Can you work these out from the model? Positions are in its coordinate system, mm. A direction names the side the tool comes from. Round coordinates to 2 decimals unless told otherwise and drop trailing zeros. Loops run counter-clockwise (first coordinate to the right, second up) from the corner with the lowest first, then second, coordinate; pieces in that order, holes last.
(1) If I drill on line 1 along Y through (x, z) = (-45, 27.75); line 2 along Y through (x, z) = (687, 2.5), over which ranges is the centre line in solid material (lowest first)?
(2) I want a section at B-B on z = 13.5. Write out the boundary of the cut face in (x, y).
(3) Will these pins go through, and if not, where does the flat tip stop? pin 1 Ø2 at (x, y) = (-8.5, 22.5) entering from +Z; pin 2 Ø0.6 at (y, z) = (40, 0.5) entering from -X; pin 3 Ø1.6 at (y, z) = (39, 0.5) entering from +X.
(4) Which directions (+Z, -Z, +X, -X, +Y, -Y) give clear straight access to the entire face, cutting with the end or side of a thin tool? Please do faces 1 (the face through (10, 2, 17)), 2 (the face through (-750, 1.6, 8.4)).
(5) I want a section at A-A on x = -250. Write out the boundary of the cut face in (y, z) (3 decimals), plus the area to 3 significant figures.
(6) I want a section at C-C on x = 462. Write out the boundary of the cut face in (y, z) (3 decimals), plus the area to 3 significant figures.
Autodesk Inventor part; units mm, degrees
ref_plane "YZ Plane" through (0, 0, 0) normal (1, 0, 0) x (0, 1, 0)
ref_plane "XZ Plane" through (0, 0, 0) normal (0, 1, 0) x (-1, 0, 0)
ref_plane "XY Plane" through (0, 0, 0) normal (0, 0, 1) x (1, 0, 0)
sketch "Sketch1" plane through (0, 0, 0) normal (0, 0, 1) x (1, 0, 0)
  line L0 (-750, 51.765) -> (750, 51.765)
  line L1 (750, 51.765) -> (750, 0)
  line L2 (750, 0) -> (-750, 0)
  line L3 (-750, 0) -> (-750, 51.765)
  point P0 (0, 0)
  point P1 (0, 0)
  dimension "d0" = 1500
  dimension "d1" = 51.765
extrude "Plate1" add sketch "Sketch1" along normal blind 2
sketch "Sketch2" plane through (750, 2, 0) normal (0, -1, 0) x (1, 0, 0)
  line L0 (-1500, 0) -> (0, 0)
  line L1 (0, 0) -> (0, 30)
  line L2 (0, 30) -> (-1500, 30)
  line L3 (-1500, 30) -> (-1500, 0)
edge flange "Flange1" height 30 angle 90 thickness 2 bend radius 2.75 thickness toward (0, -1, 0) relief round relief width 2 relief depth 1 edges at (0, 0, 2) wall of the first edge with corners at (-750, 2, 0) (750, 2, 0) (750, 2, 30) (-750, 2, 30)
bend "Bend1"
corner "Corner1"
sketch "Sketch5" plane through (0, 0, 0) normal (0, 0, -1) x (-1, 0, 0)
  line L0 (750, 51.765) -> (-750, 51.765)
  line L1 (-1, 30) -> (-1, 51.765)
  line L2 (750, 0) -> (-750, 0)
  line L3 (-1, 30) -> (1, 30)
  line L4 (1, 30) -> (1, 51.765)
  point P0 (0, 0)
  point P1 (0, 30)
  point P2 (0, 0)
  dimension "d27" = 2
  dimension "d29" = 30
extrude "Extrusion1" cut sketch "Sketch5" against normal through all
pattern_linear "Rectangular Pattern1" count 3 spacing 500 along (1, 0, 0) of "Extrusion1" first direction both ways yes
sketch "Sketch6" plane through (0, 0, 0) normal (0, 0, -1) x (-1, 0, 0)
  line L0 (-750, 51.765) -> (-750, 4.75)
  circle A0 centre (-750, 51.765) radius 22.5
  line L1 (-750, 51.765) -> (750, 51.765)
  line L2 (-499, 30) -> (-501, 30) construction
  line L3 (-499, 30) -> (-1, 30) construction
  line L4 (-1, 30) -> (-1, 51.765) construction
  line L5 (-1, 51.765) -> (-499, 51.765)
  circle A1 centre (-250, 51.765) radius 22.5
  point P0 (0, 0)
  point P1 (-727.5, 51.765)
  point P2 (-750, 29.265)
  point P3 (-250, 30)
  point P4 (-227.5, 51.765)
  point P5 (-272.5, 51.765)
  dimension "d24" = 45
extrude "Extrusion2" cut sketch "Sketch6" against normal through all contours L1 A0 L0 | L1 A1 picked at (-748.3311, 36.953) picked at (-248.2369, 40.8343)
mirror "Mirror1" about plane through (0, 0, 0) normal (1, 0, 0) of "Extrusion2"
sketch "Sketch7" plane through (0, 0, 2) normal (0, 0, 1) x (1, 0, 0)
  arc A0 (-750, 29.265) -> (-727.5, 51.765) centre (-750, 51.765) ccw
  line L0 (-750, 4.75) -> (-750, 29.265)
  line L1 (-750, 4.75) -> (750, 4.75)
  line L2 (750, 29.265) -> (750, 4.75)
  arc A1 (727.5, 51.765) -> (750, 29.265) centre (750, 51.765) ccw
  line L3 (501, 51.765) -> (727.5, 51.765)
  line L4 (501, 51.765) -> (501, 30)
  line L5 (501, 30) -> (499, 30)
  line L6 (499, 30) -> (499, 51.765)
  line L7 (1, 51.765) -> (227.5, 51.765)
  line L8 (1, 51.765) -> (1, 30)
  line L9 (1, 30) -> (-1, 30)
  line L10 (-1, 30) -> (-1, 51.765)
  line L11 (-499, 51.765) -> (-272.5, 51.765)
  line L12 (-499, 51.765) -> (-499, 30)
  line L13 (-499, 30) -> (-501, 30)
  line L14 (-501, 30) -> (-501, 51.765)
  line L15 (-727.5, 51.765) -> (-501, 51.765)
  line L16 (649, 50.765) -> (651, 50.765)
  line L17 (651, 50.765) -> (651, 51.765)
  line L18 (651, 51.765) -> (649, 51.765)
  line L19 (649, 51.765) -> (649, 50.765)
  line L20 (650, 4.75) -> (650, 51.765) construction
  line L21 (272.5, 51.765) -> (499, 51.765)
  arc A2 (227.5, 51.765) -> (272.5, 51.765) centre (250, 51.765) ccw
  line L22 (-227.5, 51.765) -> (-1, 51.765)
  arc A3 (-272.5, 51.765) -> (-227.5, 51.765) centre (-250, 51.765) ccw
  point P0 (0, 0)
  point P1 (650, 50.765)
  point P2 (649, 51.265)
  point P3 (650, 28.2575)
  dimension "d30" = 2
  dimension "d31" = 1
  dimension "d33" = 100
extrude "Extrusion3" [suppressed]
mirror "Mirror2" [suppressed]
sketch "Sketch9" plane through (0, 0, 2) normal (0, 0, 1) x (1, 0, 0)
  line L0 (494, 46.765) -> (494, 34.765) construction
  line L1 (494, 34.765) -> (294, 34.765) construction
  line L2 (294, 34.765) -> (294, 46.765) construction
  line L3 (294, 46.765) -> (494, 46.765) construction
  line L4 (499, 30) -> (499, 51.765)
  line L5 (1, 51.765) -> (499, 51.765)
  point P0 (0, 0)
  dimension "d38" = 200
  dimension "d39" = 12
  dimension "d42" = 5
  dimension "d43" = 5
mark "Mark3"
equation "\"d1\" = Стрингер_1"
equation "\"d27\" = d18"
equation "\"d29\" = Стрингер_глубина_паза"
equation "\"d43\" = d42"
equation "\"d2\" = Thickness"
equation "\"d3\" = BendReliefWidth"
equation "\"d4\" = BendReliefDepth"
equation "\"d5\" = MinimumRemnant"
equation "\"d6\" = TransitionRadius"
equation "\"d9\" = BendRadius"
equation "\"d10\" = CornerReliefSize"
equation "\"d11\" = GapSize"
equation "\"d12\" = JacobiRadiusSize"
equation "\"BendReliefWidth\" = Thickness"
equation "\"BendReliefDepth\" = 0.5 * Thickness"
equation "\"CornerReliefSize\" = 4 * Thickness"
equation "\"MinimumRemnant\" = 2 * Thickness"
equation "\"TransitionRadius\" = BendRadius"
equation "\"JacobiRadiusSize\" = BendRadius"
equation "\"GapSize\" = Thickness"
equation "\"d18\" = Thickness"
equation "\"qqqqqq\" = 67.35706"
properties part number "МОО 061 stringer back^" material "Stainless Steel"
Filled sheet:
1. line 1: y = 0 to 2
1. line 2: y = 0.57 to 3.17
2. outline: (-750, 0) - (750, 0) - (750, 2) - (-750, 2) - close
3. pin 1: stops at z = 2
3. pin 2: stops at x = -731.01
3. pin 3: stops at x = 732.05
4. face 1: +Z, +X, -X, +Y
4. face 2: +Z, -Z, -X, +Y, -Y
5. outline: (0, 4.75) arc R4.75 ccw to (4.75, 0) - (29.265, 0) - (29.265, 2) - (4.75, 2) arc R2.75 cw to (2, 4.75) - (2, 30) - (0, 30) - close
5. area: 111 mm2
6. outline: (0, 4.75) arc R4.75 ccw to (4.75, 0) - (51.765, 0) - (51.765, 2) - (4.75, 2) arc R2.75 cw to (2, 4.75) - (2, 30) - (0, 30) - close
6. area: 156 mm2
